Geometry: see drawing. Coordinates: mm, zero at the bounding-box minimum. Coordinates: 2 decimals unless noted, no trailing zeros. Write each loop counter-clockwise with the first axis right and the second up, starting at its lowest first coordinate (ties: lowest second). Pieces come first, ordered by that corner, then holes. Notation, with made-up numbers: (45.25, 23.25) -> (100.25, 23.25) arc R17 cw to (100.25, 52.25) -> close; hole circle Ø4 at (-31.5, 24.25). An arc over 180 degrees is marked (long way). Answer as a JSON object with one key per item and string values. Group by question number.
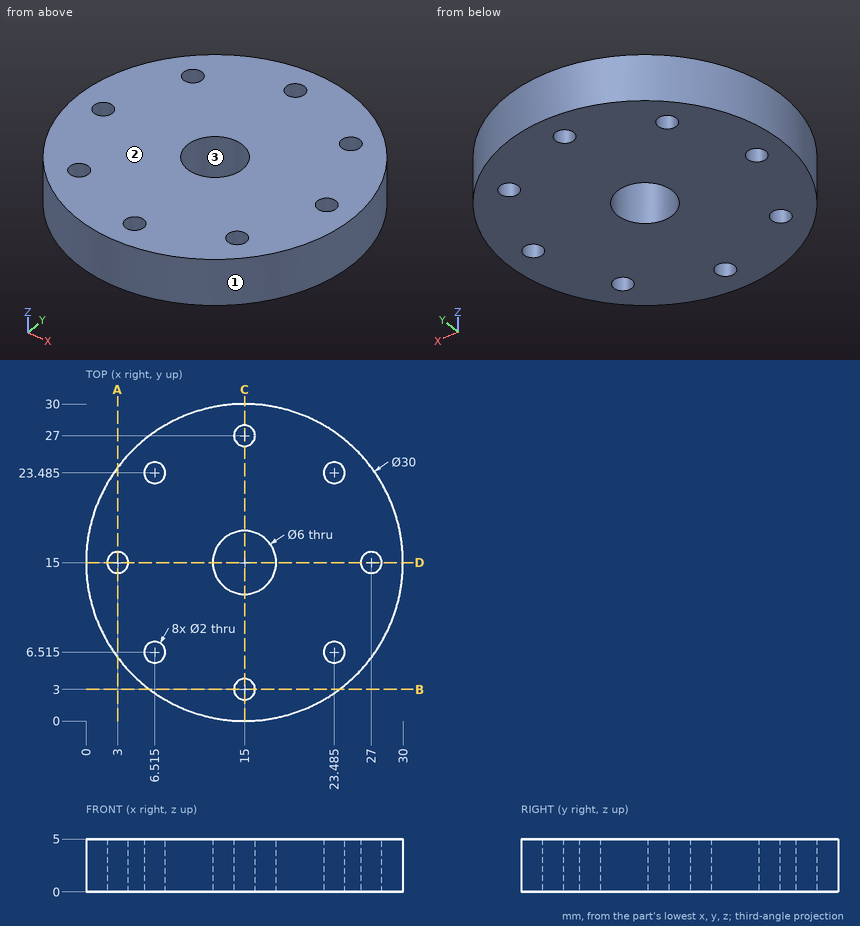
Item 1: Section A-A on x = 3. Output: boundary loops of the cut face in (y, z).
Item 2: Section C-C on x = 15. Output: boundary loops of the cut face in (y, z).
Item 3: Contact query for flat-ended pins moving along their axis: pin 1 (1.2 mm diameter, centred on x = 15, y = 27, fed in from -Z); pin 2 (1 mm diameter, centred on x = 13, z = 2.5, fed in from +Y) (1 decimal); pin 3 (3 mm diameter, centred on x = 19, z = 0.5, fed in from +Y); pin 4 (1.5 mm diameter, centred on x = 21.5, z = 3.5, fed in from +Y). Output: stop coordinate, or through.
Item 4: Ray query, L1, parallel to Y at x = 15, z = 3.55; L2, parallel to X at y = 5.75, z = 4.55; L3, parallel to Y at x = 27, z = 0.45. Return the intervals inside material, ascending. Write a range as [from, to].
Item 5: Mould query, pull axis Y, two halves, no side actions, for the marked faces 1, 2 and 3. Classes: +Y half, -Y half, draft (parallel to the pull), parting line (faces both ways), or undercut.
Answer sheet:
{
 "1": {"outline": "(6, 0) -> (14, 0) -> (14, 5) -> (6, 5) -> close; (16, 0) -> (24, 0) -> (24, 5) -> (16, 5) -> close"},
 "2": {"outline": "(0, 0) -> (2, 0) -> (2, 5) -> (0, 5) -> close; (4, 0) -> (12, 0) -> (12, 5) -> (4, 5) -> close; (18, 0) -> (26, 0) -> (26, 5) -> (18, 5) -> close; (28, 0) -> (30, 0) -> (30, 5) -> (28, 5) -> close"},
 "3": {"pin 1": "passes through", "pin 2": "stops at y = 29.9", "pin 3": "stops at y = 29.79", "pin 4": "stops at y = 28.85"},
 "4": {"L1": "y = [0, 2], [4, 12], [18, 26], [28, 30]", "L2": "x = [3.19, 5.87], [7.16, 22.84], [24.13, 26.81]", "L3": "y = [6, 14], [16, 24]"},
 "5": {"face 1": "parting line", "face 2": "draft", "face 3": "undercut"}
}
